Here's how the part is built. I have some questions about the finished solid (model axes, mm). Coordinates: 2 decimals unless noted, no trailing zeros. Write each loop counter-clockwise with the first axis right and the second up, starting at its lowest first coordinate (ties: lowest second). Pieces come first, ordered by that corner, then holes. Notation, with made-up numbers: (65, 73) -> (84, 73) arc R13 ccw to (84, 92) -> close; hole circle Ø8 at (64.25, 25). An arc over 180 degrees is marked (long way). Use a Markdown table: item, result. Add a question column.
Item 1: Imagine slicing it at C-C, the plane x = -28. Write out the boundary of the cut face in (y, z) (3 decimals), and give its area (3 significant figures).
Item 2: Imagine slicing it at B-B, the plane x = -60.5. Write out the boundary of the cut face in (y, z).
Item 3: Imagine slicing it at A-A, the plane y = 0. Write out the boundary of the cut face in (x, z), and give its area (3 significant figures).
Item 4: Imagine slicing it at D-D, the plane y = -52. Write out the boundary of the cut face in (x, z), and give its area (3 significant figures).
Item 5: If I drill on line 1 along X through (y, z) = (5, 2.5); line 2 along Y through (x, z) = (66.5, 4.75); line 3 along Y through (x, z) = (-19, 6), over which ranges is the centre line in solid material (lowest first)? Write a range as from..to.
Item 6: Will these pins go through, and if not, where does the flat tip stop? pin 1 Ø2.5 at (x, z) = (64.5, 3) entering from +Y; pin 2 Ø2.5 at (x, z) = (-49, 5.5) entering from +Y; pin 3 Ø4 at (x, z) = (-64, 4.5) entering from -Y.
Item 7: If we mould it in two halves opening along X, with no side actions, what happens to faces 1 (the flat face through (-46.626, 34.252, 3.757)), 2 (the flat face through (-1, 1, 0))? For each: pulls with the +X half, pulls with the -X half, needs draft (parallel to the pull), parting line crosses it, or undercut.
```python
from build123d import *

# Parameters (mm, degrees)
SKETCH1_R           = 95.25
BOSS_EXTRUDE1_DEPTH = 7.62


with BuildPart() as part:
    # Sketch1 → Boss-Extrude1 (new body)
    with BuildSketch(Plane.XY):
        Circle(SKETCH1_R)
        with BuildLine():
            Line((-6.35, 82.55), (-6.35, 31.75))
            ThreePointArc((-6.35, 31.75), (0, 25.4), (6.35, 31.75))
            Line((6.35, 31.75), (6.35, 82.55))
            ThreePointArc((6.35, 82.55), (0, 88.9), (-6.35, 82.55))
        make_face(mode=Mode.SUBTRACT)
        with BuildLine():
            Line((46.774261314, 68.315397082), (21.374261314, 24.32130657))
            ThreePointArc((21.374261314, 24.32130657), (12.7, 21.997045256), (10.375738686, 30.67130657))
            Line((10.375738686, 30.67130657), (35.775738686, 74.665397082))
            ThreePointArc((35.775738686, 74.665397082), (44.45, 76.989658396), (46.774261314, 68.315397082))
        make_face(mode=Mode.SUBTRACT)
        with BuildLine():
            Line((74.665397082, 35.775738686), (30.67130657, 10.375738686))
            ThreePointArc((30.67130657, 10.375738686), (21.997045256, 12.7), (24.32130657, 21.374261314))
            Line((24.32130657, 21.374261314), (68.315397082, 46.774261314))
            ThreePointArc((68.315397082, 46.774261314), (76.989658396, 44.45), (74.665397082, 35.775738686))
        make_face(mode=Mode.SUBTRACT)
        with BuildLine():
            Line((82.55, -6.35), (31.75, -6.35))
            ThreePointArc((31.75, -6.35), (25.4, 0), (31.75, 6.35))
            Line((31.75, 6.35), (82.55, 6.35))
            ThreePointArc((82.55, 6.35), (88.9, 0), (82.55, -6.35))
        make_face(mode=Mode.SUBTRACT)
        with BuildLine():
            Line((68.315397082, -46.774261314), (24.32130657, -21.374261314))
            ThreePointArc((24.32130657, -21.374261314), (21.997045256, -12.7), (30.67130657, -10.375738686))
            Line((30.67130657, -10.375738686), (74.665397082, -35.775738686))
            ThreePointArc((74.665397082, -35.775738686), (76.989658396, -44.45), (68.315397082, -46.774261314))
        make_face(mode=Mode.SUBTRACT)
        with BuildLine():
            Line((35.775738686, -74.665397082), (10.375738686, -30.67130657))
            ThreePointArc((10.375738686, -30.67130657), (12.7, -21.997045256), (21.374261314, -24.32130657))
            Line((21.374261314, -24.32130657), (46.774261314, -68.315397082))
            ThreePointArc((46.774261314, -68.315397082), (44.45, -76.989658396), (35.775738686, -74.665397082))
        make_face(mode=Mode.SUBTRACT)
        with BuildLine():
            Line((-6.35, -82.55), (-6.35, -31.75))
            ThreePointArc((-6.35, -31.75), (0, -25.4), (6.35, -31.75))
            Line((6.35, -31.75), (6.35, -82.55))
            ThreePointArc((6.35, -82.55), (0, -88.9), (-6.35, -82.55))
        make_face(mode=Mode.SUBTRACT)
        with BuildLine():
            Line((-46.774261314, -68.315397082), (-21.374261314, -24.32130657))
            ThreePointArc((-21.374261314, -24.32130657), (-12.7, -21.997045256), (-10.375738686, -30.67130657))
            Line((-10.375738686, -30.67130657), (-35.775738686, -74.665397082))
            ThreePointArc((-35.775738686, -74.665397082), (-44.45, -76.989658396), (-46.774261314, -68.315397082))
        make_face(mode=Mode.SUBTRACT)
        with BuildLine():
            Line((-74.665397082, -35.775738686), (-30.67130657, -10.375738686))
            ThreePointArc((-30.67130657, -10.375738686), (-21.997045256, -12.7), (-24.32130657, -21.374261314))
            Line((-24.32130657, -21.374261314), (-68.315397082, -46.774261314))
            ThreePointArc((-68.315397082, -46.774261314), (-76.989658396, -44.45), (-74.665397082, -35.775738686))
        make_face(mode=Mode.SUBTRACT)
        with BuildLine():
            Line((-82.55, 6.35), (-31.75, 6.35))
            ThreePointArc((-31.75, 6.35), (-25.4, 0), (-31.75, -6.35))
            Line((-31.75, -6.35), (-82.55, -6.35))
            ThreePointArc((-82.55, -6.35), (-88.9, 0), (-82.55, 6.35))
        make_face(mode=Mode.SUBTRACT)
        with BuildLine():
            Line((-68.315397082, 46.774261314), (-24.32130657, 21.374261314))
            ThreePointArc((-24.32130657, 21.374261314), (-21.997045256, 12.7), (-30.67130657, 10.375738686))
            Line((-30.67130657, 10.375738686), (-74.665397082, 35.775738686))
            ThreePointArc((-74.665397082, 35.775738686), (-76.989658396, 44.45), (-68.315397082, 46.774261314))
        make_face(mode=Mode.SUBTRACT)
        with BuildLine():
            Line((-35.775738686, 74.665397082), (-10.375738686, 30.67130657))
            ThreePointArc((-10.375738686, 30.67130657), (-12.7, 21.997045256), (-21.374261314, 24.32130657))
            Line((-21.374261314, 24.32130657), (-46.774261314, 68.315397082))
            ThreePointArc((-46.774261314, 68.315397082), (-44.45, 76.989658396), (-35.775738686, 74.665397082))
        make_face(mode=Mode.SUBTRACT)
    extrude(amount=BOSS_EXTRUDE1_DEPTH)


solid = part.part
```
Ans:
| question | item | result |
|---|---|---|
| 1 | outline | (-91.042, 0) -> (-61.197, 0) -> (-61.197, 7.62) -> (-91.042, 7.62) -> close; (-35.797, 0) -> (-23.498, 0) -> (-23.498, 7.62) -> (-35.797, 7.62) -> close; (-9.545, 0) -> (-5.124, 0) -> (-5.124, 7.62) -> (-9.545, 7.62) -> close; (5.124, 0) -> (9.545, 0) -> (9.545, 7.62) -> (5.124, 7.62) -> close; (23.498, 0) -> (35.797, 0) -> (35.797, 7.62) -> (23.498, 7.62) -> close; (61.197, 0) -> (91.042, 0) -> (91.042, 7.62) -> (61.197, 7.62) -> close |
| 1 | area | 710 mm^2 |
| 2 | outline | (-73.57, 0) -> (-42.26, 0) -> (-42.26, 7.62) -> (-73.57, 7.62) -> close; (-27.6, 0) -> (-6.35, 0) -> (-6.35, 7.62) -> (-27.6, 7.62) -> close; (6.35, 0) -> (27.6, 0) -> (27.6, 7.62) -> (6.35, 7.62) -> close; (42.26, 0) -> (73.57, 0) -> (73.57, 7.62) -> (42.26, 7.62) -> close |
| 3 | outline | (-95.25, 0) -> (-88.9, 0) -> (-88.9, 7.62) -> (-95.25, 7.62) -> close; (-25.4, 0) -> (25.4, 0) -> (25.4, 7.62) -> (-25.4, 7.62) -> close; (88.9, 0) -> (95.25, 0) -> (95.25, 7.62) -> (88.9, 7.62) -> close |
| 3 | area | 484 mm^2 |
| 4 | outline | (-79.8, 0) -> (-37.35, 0) -> (-37.35, 7.62) -> (-79.8, 7.62) -> close; (-22.69, 0) -> (-6.35, 0) -> (-6.35, 7.62) -> (-22.69, 7.62) -> close; (6.35, 0) -> (22.69, 0) -> (22.69, 7.62) -> (6.35, 7.62) -> close; (37.35, 0) -> (79.8, 0) -> (79.8, 7.62) -> (37.35, 7.62) -> close |
| 4 | area | 896 mm^2 |
| 5 | line 1 | x = -95.12..-86.46, -27.84..27.84, 86.46..95.12 |
| 5 | line 2 | y = -68.19..-45.73, -31.06..-6.35, 6.35..31.06, 45.73..68.19 |
| 5 | line 3 | y = -93.34..-45.61, -21.97..21.97, 45.61..93.34 |
| 6 | pin 1 | stops at y = 71.22 |
| 6 | pin 2 | stops at y = 82.42 |
| 6 | pin 3 | stops at y = -72.31 |
| 7 | face 1 | undercut |
| 7 | face 2 | needs draft |
